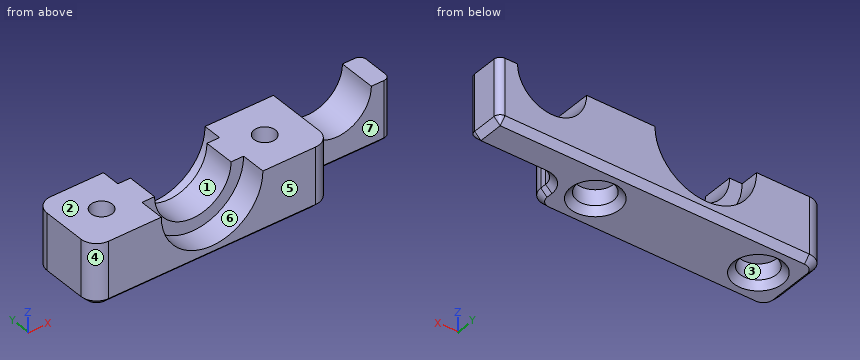
from build123d import *

# Parameters (mm, degrees)
F1_DEPTH      = 6
F2_DEPTH      = 2
F2_DEPTH_BACK = 3
F3_DEPTH      = 6
F4_R          = 2.9
F4_R_2        = 1.7
F5_DEPTH      = 3.5
F6_R          = 2.5
F7_T4_DEPTH   = 10
F7_S5_R       = 5.5
F7_T6_DEPTH   = 7
F7_T7_DEPTH   = 22.5
F8_R          = 1
F9_T1_DEPTH   = 48.4999999995
F9_T3_DEPTH   = 10.5
F9_T5_DEPTH   = 4
F9_T7_DEPTH   = 1
F9_T9_DEPTH   = 32.9999999994
F9_T11_DEPTH  = 7
F9_T18_ANGLE  = 90
F9_T20_ANGLE  = 89.9999999974
F9_T22_ANGLE  = 90
F9_T24_ANGLE  = 90.0000000053
F9_T26_ANGLE  = 90
F9_T28_ANGLE  = 90
F10_R         = 1.7
F11_DEPTH     = 6.4


# Not quite as in the source:
# - a fillet or chamfer that OpenCascade refuses, or shapes differently, is made with other operations: its cross-section is extruded or revolved along the edge and cut away or added


with BuildPart() as f1:
    # F0 (on Front) → F1 (new body, symmetric)
    with BuildSketch(Plane.XZ):
        with BuildLine():
            Line((18.9999999997, 0), (18.9999999997, 10))
            Line((18.9999999997, 10), (8.099, 10))
            ThreePointArc((8.099, 10), (0, 1.901), (-8.099, 10))
            Line((-8.099, 10), (-18.9999999997, 10))
            Line((-18.9999999997, 10), (-18.9999999997, 0))
            Line((-18.9999999997, 0), (18.9999999997, 0))
        make_face()
    extrude(amount=F1_DEPTH, both=True)

    # F0 (on Front) → F2 (join, two sides)
    with BuildSketch(Plane.XZ) as f2_sk:
        with BuildLine():
            ThreePointArc((-8.099, 10), (0, 1.901), (8.099, 10))
            Line((8.099, 10), (6.099, 10))
            ThreePointArc((6.099, 10), (0, 3.901), (-6.099, 10))
            Line((-6.099, 10), (-8.099, 10))
        make_face()
    extrude(amount=F2_DEPTH)
    extrude(f2_sk.sketch, amount=-F2_DEPTH_BACK)

    # F0 (on Front) → F3 (join)
    with BuildSketch(Plane.XZ):
        with BuildLine():
            ThreePointArc((29.9999999997, 10), (24.4999999997, 4.5), (18.9999999997, 10))
            Line((18.9999999997, 10), (18.9999999997, 0))
            Line((18.9999999997, 0), (32.9999999997, 0))
            Line((32.9999999997, 0), (32.9999999997, 10))
            Line((32.9999999997, 10), (29.9999999997, 10))
        make_face()
    extrude(amount=-F3_DEPTH)

    # F4 (on face) → F5 (cut)
    with BuildSketch(Plane(origin=(0, 0, 0), x_dir=(1, 0, 0), z_dir=(0, 0, -1))):
        with Locations((13, 0)):
            Circle(F4_R)
        with Locations((13, 0)):
            Circle(F4_R_2, mode=Mode.SUBTRACT)
        with Locations((-13, 0)):
            Circle(F4_R)
        with Locations((-13, 0)):
            Circle(F4_R_2, mode=Mode.SUBTRACT)
        with Locations((13, 0)):
            Circle(F4_R_2)
        with Locations((-13, 0)):
            Circle(F4_R_2)
    extrude(amount=-F5_DEPTH, mode=Mode.SUBTRACT)

    # F6
    f6_edges = [f1.edges().sort_by_distance(p)[0] for p in [
        (-19, 6, 5),
        (-19, -6, 5),
    ]]
    fillet(f6_edges, radius=F6_R)

    # F7: fillet of radius 2.5 on 2 edges, made by hand


with BuildPart() as f7_tool2:
    # F7_s3 → F7_t4 (new body)
    with BuildSketch(Plane.XY.offset(10)):
        with BuildLine():
            ThreePointArc((21.4999999997, 0), (19.7322330468, -0.732233047), (18.9999999997, -2.5))
            Line((18.9999999997, -2.5), (18.9999999997, 0))
            Line((18.9999999997, 0), (21.4999999997, 0))
        make_face()
    extrude(amount=-F7_T4_DEPTH)

    # F7_s5 → F7_t6 (cut, symmetric)
    with BuildSketch(Plane.XZ.offset(1.2)):
        with Locations((24.4999999997, 10)):
            Circle(F7_S5_R)
    extrude(amount=F7_T6_DEPTH, both=True, mode=Mode.SUBTRACT)


with BuildPart() as f1_1:
    add(f1.part)

    # F7_t1: union F7_tool2
    add(f7_tool2.part)

    # F7_s8 → F7_t7 (cut)
    with BuildSketch(Plane.XY.offset(-6.25)):
        with BuildLine():
            ThreePointArc((16.4999999997, -6), (18.2677669527, -5.267766953), (18.9999999997, -3.5))
            Line((18.9999999997, -3.5), (18.9999999997, -6))
            Line((18.9999999997, -6), (16.4999999997, -6))
        make_face()
    extrude(amount=F7_T7_DEPTH, mode=Mode.SUBTRACT)

    # F8
    f8_edges = [f1_1.edges().sort_by_distance(p)[0] for p in [
        (33, 6, 5),
        (33, 0, 5),
    ]]
    fillet(f8_edges, radius=F8_R)

    # F9: chamfer of 1 on 14 edges, made by hand

    # F9_s2 → F9_t1 (cut)
    with BuildSketch(Plane.YZ.offset(-16.4999999997)):
        Polygon((5, 0), (6, 1), (6, 0), align=None)
    extrude(amount=F9_T1_DEPTH, mode=Mode.SUBTRACT)

    # F9_s4 → F9_t3 (cut)
    with BuildSketch(Plane.YZ.offset(21.4999999997)):
        Polygon((1, 0), (0, 1), (0, 0), align=None)
    extrude(amount=F9_T3_DEPTH, mode=Mode.SUBTRACT)

    # F9_s6 → F9_t5 (cut)
    with BuildSketch(Plane.XZ.offset(-5)):
        Polygon((31.9999999997, 0), (32.9999999997, 1), (32.9999999997, 0), align=None)
    extrude(amount=F9_T5_DEPTH, mode=Mode.SUBTRACT)

    # F9_s8 → F9_t7 (cut)
    with BuildSketch(Plane.XZ.offset(2.5)):
        Polygon((17.9999999997, 0), (18.9999999997, 1), (18.9999999997, 0), align=None)
    extrude(amount=F9_T7_DEPTH, mode=Mode.SUBTRACT)

    # F9_s10 → F9_t9 (cut)
    with BuildSketch(Plane.YZ.offset(-16.4999999997)):
        Polygon((-5, 0), (-6, 1), (-6, 0), align=None)
    extrude(amount=F9_T9_DEPTH, mode=Mode.SUBTRACT)

    # F9_s12 → F9_t11 (cut)
    with BuildSketch(Plane.XZ.offset(-3.5)):
        Polygon((-17.9999999997, 0), (-18.9999999997, 1), (-18.9999999997, 0), align=None)
    extrude(amount=F9_T11_DEPTH, mode=Mode.SUBTRACT)

    # F9_s13 → F9_t14 (revolve, cut)
    with BuildSketch(Plane.XZ):
        Polygon((-9.1, 0), (-10.1, 1), (-10.1, 0), align=None)
    revolve(axis=Axis((-13, 0, 0), (0, 0, -1)), mode=Mode.SUBTRACT)

    # F9_s15 → F9_t16 (revolve, cut)
    with BuildSketch(Plane.XZ):
        Polygon((16.9, 0), (15.9, 1), (15.9, 0), align=None)
    revolve(axis=Axis((13, 0, 0), (0, 0, -1)), mode=Mode.SUBTRACT)

    # F9_s17 → F9_t18 (revolve, cut)
    with BuildSketch(Plane.YZ.offset(31.9999999997)):
        Polygon((1, 0), (0, 1), (0, 0), align=None)
    revolve(axis=Axis((31.9999999997, 1, 0), (0, 0, 1)), revolution_arc=F9_T18_ANGLE, mode=Mode.SUBTRACT)

    # F9_s19 → F9_t20 (revolve, cut)
    with BuildSketch(Plane.YZ.offset(21.4999999998)):
        Polygon((1, 0), (0, 1), (0, 0), align=None)
    revolve(axis=Axis((21.4999999998, -2.5000000001, 0), (0, 0, 1)), revolution_arc=F9_T20_ANGLE, mode=Mode.SUBTRACT)

    # F9_s21 → F9_t22 (revolve, cut)
    with BuildSketch(Plane.XZ.offset(-5)):
        Polygon((31.9999999997, 0), (32.9999999997, 1), (32.9999999997, 0), align=None)
    revolve(axis=Axis((31.9999999997, 5, 0), (0, 0, 1)), revolution_arc=F9_T22_ANGLE, mode=Mode.SUBTRACT)

    # F9_s23 → F9_t24 (revolve, cut)
    with BuildSketch(Plane.XZ.offset(3.5000000001)):
        Polygon((17.9999999997, 0), (18.9999999997, 1), (18.9999999997, 0), align=None)
    revolve(axis=Axis((16.4999999998, -3.5000000001, 0), (0, 0, -1)), revolution_arc=F9_T24_ANGLE, mode=Mode.SUBTRACT)

    # F9_s25 → F9_t26 (revolve, cut)
    with BuildSketch(Plane.YZ.offset(-16.4999999997)):
        Polygon((5, 0), (6, 1), (6, 0), align=None)
    revolve(axis=Axis((-16.4999999997, 3.5, 0), (0, 0, 1)), revolution_arc=F9_T26_ANGLE, mode=Mode.SUBTRACT)

    # F9_s27 → F9_t28 (revolve, cut)
    with BuildSketch(Plane.XZ.offset(3.5)):
        Polygon((-17.9999999997, 0), (-18.9999999997, 1), (-18.9999999997, 0), align=None)
    revolve(axis=Axis((-16.4999999997, -3.5, 0), (0, 0, 1)), revolution_arc=F9_T28_ANGLE, mode=Mode.SUBTRACT)

    # F10 (on face) → F11 (cut)
    with BuildSketch(Plane.XY.offset(10)):
        with Locations((-13, 0)):
            Circle(F10_R)
        with Locations((13, 0)):
            Circle(F10_R)
    extrude(amount=-F11_DEPTH, mode=Mode.SUBTRACT)


solid = f1_1.part
Geometry check sheet. Reference: the model listing, model coordinates, mm. Face numbers are marked on the shaded views. A direction names the side the tool comes from. Give positions to 0.01 mm unless a question says otherwise; leave off trailing zeros. Order: outer loops, then holes, each group sorted by start corner. A loop starts at its lowest first (then second) coordinate and runs counter-clockwise, first axis right, second up.
1) Cross-section at B-B (x = 0). Record the boundary of the cut face in (y, z).
Results are:
outline: (-6, 1) - (-5, 0) - (5, 0) - (6, 1) - (6, 1.9) - (3, 1.9) - (3, 3.9) - (-2, 3.9) - (-2, 1.9) - (-6, 1.9) - close
2) Cross-section at D-D (x = 13). Record the boundary of the cut face in (y, z), then the cut area to 3 significant figures.
Results are:
outline: (-6, 1) - (-5, 0) - (-3.9, 0) - (-2.9, 1) - (-2.9, 3.5) - (2.9, 3.5) - (2.9, 1) - (3.9, 0) - (5, 0) - (6, 1) - (6, 10) - (1.7, 10) - (1.7, 3.6) - (-1.7, 3.6) - (-1.7, 10) - (-6, 10) - close
area: 75.9 mm2
3) Draft check along X on the marked faces 1, 2, 3 and 4. Enter one of: released by +X, released by -X, zero draft, split by the parting line, or undercut.
Results are:
face 1: undercut
face 2: zero draft
face 3: undercut
face 4: released by -X
4) Cross-section at C-C (z = 2.5). Record the boundary of the cut face in (x, y), then the cut area to 3 significant figures.
Results are:
outline: (-19, -3.5) arc R2.5 ccw to (-16.5, -6) - (-3.06, -6) - (-3.06, -2) - (3.06, -2) - (3.06, -6) - (16.5, -6) arc R2.5 ccw to (19, -3.5) - (19, -2.5) arc R2.5 cw to (21.5, 0) - (32, 0) arc R1 ccw to (33, 1) - (33, 5) arc R1 ccw to (32, 6) - (3.06, 6) - (3.06, 3) - (-3.06, 3) - (-3.06, 6) - (-16.5, 6) arc R2.5 ccw to (-19, 3.5) - close; hole circle Ø5.8 at (-13, 0); hole circle Ø5.8 at (13, 0)
area: 441 mm2
5) Material ranges on probe 1 along Y at (x, z) = (13, 6.5); probe 2 along Y at (x, z) = (13, 2.1); probe 3 along X at (y, z) = (1, 1.5), recorded low to high.
Results are:
probe 1: y = -6 to -1.7, 1.7 to 6
probe 2: y = -6 to -2.9, 2.9 to 6
probe 3: x = -19 to -15.72, -10.28 to 10.28, 15.72 to 33
6) Cross-section at A-A (z = 6). Give the number of separate pieces and of enclosed holes in the cut face, then the cut area to 3 significant figures.
Results are:
separate pieces: 3
enclosed holes: 2
area: 329 mm2
7) Gauge pin test, flat ends, axial feed: pin 1 (4.5 mm diameter, centred on x = -13, y = 0, fed in from -Z); pin 2 (4.5 mm diameter, centred on x = 12, y = 0.5, fed in from -Z); pin 3 (0.5 mm diameter, centred on y = -3, z = 7.5, fed in from +X). Record the tip position at first contact, or that the pin passes through.
Results are:
pin 1: stops at z = 3.5
pin 2: stops at z = 0.53
pin 3: stops at x = 19
8) Tool access check on the marked faces 5, 6 and 7. Record the directions out of +Z, -Z, +X, -X, +Y, -Y that give a thin tool (end or side, any length) a straight path to the whole face; none if there is none.
Results are:
face 5: +Z, -Z, +X, -X, -Y
face 6: +Z, -Y
face 7: +Z, -Z, +X, -Y
